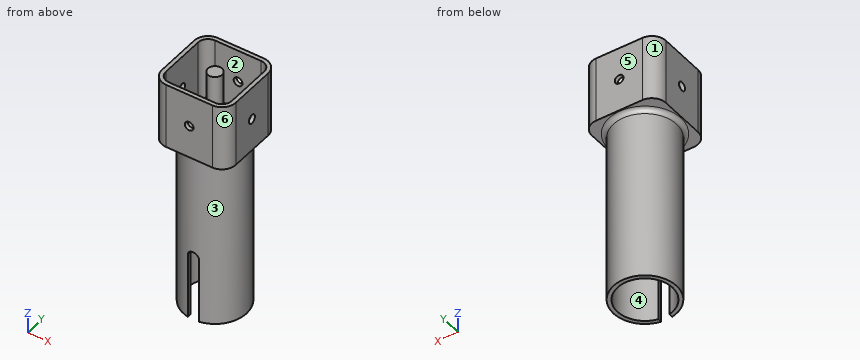
```python
from build123d import *

# Parameters (mm, degrees)
SKETCH_1_R               = 3.25
EXTRUDE_1_DEPTH          = 30
SHELL_1_T                = -1.8
SKETCH_1_3_R             = 3.25
EXTRUDE_2_DEPTH          = 30
CUT_EXTRUDE_1_REACH      = 50.075
SKETCH_2_R               = 2
PATTERN_CIRCULAR_1_COUNT = 4
SKETCH_3_R               = 14.3
SKETCH_3_R_2             = 12.5
EXTRUDE_3_DEPTH          = 80
CUT_EXTRUDE_2_REACH      = 85.453
CUT_EXTRUDE_2_END_RADIUS = 14.3
FILLET_1_R               = 2


with BuildPart() as part:
    # 草圖1 → 填料-伸長1 (new body)
    with BuildSketch(Plane.XY):
        with BuildLine():
            Line((10.5, 16.8), (-10.5, 16.8))
            ThreePointArc((-10.5, 16.8), (-14.954772721, 14.954772721), (-16.8, 10.5))
            Line((-16.8, 10.5), (-16.8, -10.5))
            ThreePointArc((-16.8, -10.5), (-14.954772721, -14.954772721), (-10.5, -16.8))
            Line((-10.5, -16.8), (10.5, -16.8))
            ThreePointArc((10.5, -16.8), (14.954772721, -14.954772721), (16.8, -10.5))
            Line((16.8, -10.5), (16.8, 10.5))
            ThreePointArc((16.8, 10.5), (14.954772721, 14.954772721), (10.5, 16.8))
        make_face()
        Circle(SKETCH_1_R, mode=Mode.SUBTRACT)
        Circle(SKETCH_1_R)
    extrude(amount=EXTRUDE_1_DEPTH)

    # 薄殼1
    shell_1_openings = [part.faces().sort_by_distance(p)[0] for p in [
        (0, 0, 30),
    ]]
    offset(amount=SHELL_1_T, openings=shell_1_openings, kind=Kind.INTERSECTION)

    # 草圖1<3> → 填料-伸長2 (add)
    with BuildSketch(Plane.XY):
        Circle(SKETCH_1_3_R)
    extrude(amount=EXTRUDE_2_DEPTH)

    # 草圖2 → 除料-伸長1 (cut, up to next)
    with BuildSketch(Plane(origin=(0, 16.8, 0), x_dir=(1, 0, 0), z_dir=(0, 1, 0)), mode=Mode.PRIVATE) as cut_extrude_1_sk1:
        with Locations(Location((0, -15, 0), (0, 0, 270))):
            Circle(SKETCH_2_R)
    cut_extrude_1_tool1 = extrude(cut_extrude_1_sk1.sketch, amount=-CUT_EXTRUDE_1_REACH, mode=Mode.PRIVATE) & part.part
    cut_extrude_1 = cut_extrude_1_tool1.solids().sort_by_distance((0, 16.8, 15))[0]
    add(cut_extrude_1, mode=Mode.SUBTRACT)

    # 環狀複製排列1: 除料-伸長1 ×4 about axis
    pattern_circular_1_axis = Axis((0, 0, 30), (0, 0, -1))
    for i in range(1, PATTERN_CIRCULAR_1_COUNT):
        add(cut_extrude_1.rotate(pattern_circular_1_axis, i * 360 / PATTERN_CIRCULAR_1_COUNT), mode=Mode.SUBTRACT)

    # 草圖3 → 填料-伸長3 (add)
    with BuildSketch(Plane(origin=(0, 0, 0), x_dir=(-1, 0, 0), z_dir=(0, 0, -1))):
        with Locations(Location((0, 0, 0), (0, 0, 180))):
            Circle(SKETCH_3_R)
        Circle(SKETCH_3_R_2, mode=Mode.SUBTRACT)
    extrude(amount=EXTRUDE_3_DEPTH)

    # 除料-伸長2: up to this cylinder (the profile starts inside it)
    cut_extrude_2_end = Plane(origin=(0, 0, -65.346562), z_dir=(0, 0, 1)) * Cylinder(CUT_EXTRUDE_2_END_RADIUS, 200.506, mode=Mode.PRIVATE)
    # 草圖4 → 除料-伸長2 (cut, up to the surface)
    with BuildSketch(Plane(origin=(0, 0, 0), x_dir=(1, 0, 0), z_dir=(0, 1, 0)), mode=Mode.PRIVATE) as cut_extrude_2_sk1:
        with BuildLine():
            Line((-2.5, 82.665609903), (2.5, 82.665609903))
            Line((2.5, 82.665609903), (2.5, 50))
            ThreePointArc((2.5, 50), (0, 47.5), (-2.5, 50))
            Line((-2.5, 50), (-2.5, 82.665609903))
        make_face()
    cut_extrude_2_tool1 = extrude(cut_extrude_2_sk1.sketch, amount=-CUT_EXTRUDE_2_REACH, mode=Mode.PRIVATE) & cut_extrude_2_end
    add(cut_extrude_2_tool1.solids().sort_by_distance((0, 0, -65.346562))[0], mode=Mode.SUBTRACT)

    # 圓角1
    fillet_1_edges = [part.edges().sort_by_distance(p)[0] for p in [
        (-14.3, 0, 0),
    ]]
    fillet(fillet_1_edges, radius=FILLET_1_R)


solid = part.part
```
Model file for the job. Use its own axes, mm. Face numbers are marked on the shaded views. A direction names the side the tool comes from. Coordinates: 2 decimals unless noted, no trailing zeros. Order: outer loops, then holes, each group sorted by start corner. A loop starts at its lowest first (then second) coordinate and runs counter-clockwise, first axis right, second up. Notation, with made-up numbers: (23.25, 35.5) - (74.25, 35.5) arc R20 cw to (74.25, 55.5) - close; hole circle Ø10 at (19.25, -37). An arc over 180 degrees is marked (long way). Return JSON: item names as keys, results as strings. Group by question number.
1) Probe line 1 (X direction, y = -3.5, z = 10); line 2 (Y direction, x = 0, z = -35.5). List the from-to ranges inside material, lowest first. Write a range as from..to.
2) Saw through at D-D, the plane z = -7.5. Write the cut outline in (x, y).
3) Tool access for the marked faces 1, 2 and 3: list every direction of +Z, -Z, +X, -X, +Y, -Y with a clear straight run to the whole face (end or side of a thin tool).
4) Flat gauge pins, fed straight in: P1, Ø6, axis at x = 3.5, z = -16, coming from the +Y side; P2, Ø2, axis at y = 6.5, z = -13.5, coming from the -X side; P3, Ø5, axis at x = 2.5, y = -10.5, coming from the +Z side. Where does each tip first touch, or does it go through?
5) Mould opens along X. For the marked faces 4, 5 and 6 say: released by +X, released by -X, zero draft, split by the parting line, or undercut.
6) Saw through at A-A, the plane z = 15. Count the separate pieces of the cut face and the enclosed holes in it, plus the area to 3 significant figures.
Values found:
{
 "1": {"line 1": "x = -16.8..-15, 15..16.8", "line 2": "y = -14.3..-12.5, 12.5..14.3"},
 "2": {"outline": "circle Ø28.6 at (0, 0); hole circle Ø25 at (0, 0)"},
 "3": {"face 1": "+Z, -Z, -X, +Y", "face 2": "+Z", "face 3": "-Z"},
 "4": {"P1": "stops at y = 14.29", "P2": "stops at x = -13.2", "P3": "stops at z = 1.8"},
 "5": {"face 4": "undercut", "face 5": "zero draft", "face 6": "released by +X"},
 "6": {"separate pieces": "5", "enclosed holes": "0", "area": "217 mm²"}
}
